The model under review builds one solid part; all positions refer to its coordinate system, in mm. Face numbers are marked on the shaded views. Coordinates: 2 decimals unless noted, no trailing zeros. Loops run counter-clockwise (first coordinate to the right, second up) from the corner with the lowest first, then second, coordinate; pieces in that order, holes last. Notation, with made-up numbers: M -1.5,70 L 13.5,70 A18 ccw 13.5,105 Z; hole C -9.75,-13 d1. An arc over 180 degrees is marked long. Use CSV: the item, a comma, the result in double quotes. Start each with the question number.
1. Draft analysis for pull direction Y (two halves, no side actions). For the marked faces 1, 2, 3 and 4, state which applies: +Y half, -Y half, draft (parallel to the pull), parting line (faces both ways), or undercut.
2. Clearance check with flat-ended pins moving along their axes: P1, Ø2, axis at x = 2, z = 5.5, coming from the +Y side; P2, Ø3, axis at y = -6.5, z = 1.5, coming from the +X side; P3, Ø1, axis at x = -30.5, y = 23, coming from the -Z side. State where each tip first meets the part, or that it passes through.
3. Add section A-A, the plane x = 0. Write out the cut boundary in (y, z), then the cut area to 3 significant figures.
4. Add section B-B, the plane z = 1.25. Write out the cut boundary in (x, y), then the cut area to 3 significant figures.
5. For L1, parallel to X at y = 1.5, z = 4; L2, parallel to X at y = 2, z = 5.5; L3, parallel to X at y = 23, z = 3, list the stretches that pass through material, from the lowest coordinate up.
6. Add section C-C, the plane y = 0. Write out the cut boundary in (x, z).
7. Add section D-D, the plane x = 27. Write out the cut boundary in (y, z), then the cut area to 3 significant figures.
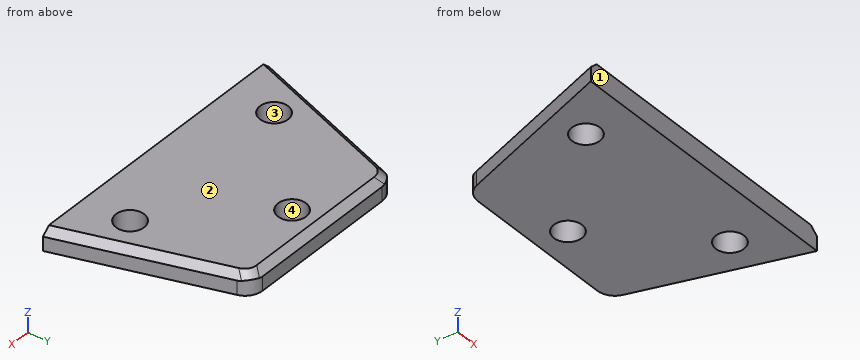
from build123d import *

# Parameters (mm, degrees)
F0_R     = 4
F1_DEPTH = 6
F2_SIZE  = 2
F3_F1_R  = 5
F3_F2_R  = 5
F3_F3_R  = 5
F3_F4_R  = 5


with BuildPart() as f1:
    # F0 (on Top) → F1 (new body)
    with BuildSketch(Plane.XY):
        Polygon((40.4508497187, -13.143277803), (25, 34.4095480118), (-25, 34.4095480118), (-40.4508497187, -13.143277803), align=None)
        with Locations((-25.7480759174, 0)):
            Circle(F0_R, mode=Mode.SUBTRACT)
        with Locations((25.7480759174, 0)):
            Circle(F0_R, mode=Mode.SUBTRACT)
        with Locations((0, 25.7480759174)):
            Circle(F0_R, mode=Mode.SUBTRACT)
    extrude(amount=F1_DEPTH)

    # F2
    f2_edges = [f1.edges().sort_by_distance(p)[0] for p in [
        (0, 34.409548, 6),
        (32.725425, 10.633135, 6),
        (-32.725425, 10.633135, 6),
    ]]
    chamfer(f2_edges, length=F2_SIZE)

    # F3: fillet of radius 5 on 4 edges, made by hand

    # F3_f1
    f3_f1_edges = [f1.edges().sort_by_distance(p)[0] for p in [
        (25, 34.4095480118, 2),
    ]]
    fillet(f3_f1_edges, radius=F3_F1_R)

    # F3_f2
    f3_f2_edges = [f1.edges().sort_by_distance(p)[0] for p in [
        (23.9265642827, 32.9320904977, 5.4774575141),
    ]]
    fillet(f3_f2_edges, radius=F3_F2_R)

    # F3_f3
    f3_f3_edges = [f1.edges().sort_by_distance(p)[0] for p in [
        (-25, 34.4095480118, 2),
    ]]
    fillet(f3_f3_edges, radius=F3_F3_R)

    # F3_f4
    f3_f4_edges = [f1.edges().sort_by_distance(p)[0] for p in [
        (-23.9265642827, 32.9320904977, 5.4774575141),
    ]]
    fillet(f3_f4_edges, radius=F3_F4_R)


solid = f1.part
Computed:
1,face 1,"-Y half"
1,face 2,"draft"
1,face 3,"undercut"
1,face 4,"undercut"
2,P1,"stops at y = 33.91"
2,P2,"stops at x = 38.78"
2,P3,"passes through"
3,outline,"M -13.14,0 L 21.75,0 L 21.75,6 L -13.14,6 Z; M 29.75,0 L 34.41,0 L 34.41,4 L 32.41,6 L 29.75,6 Z"
3,area,"235 mm^2"
4,outline,"M -40.45,-13.14 L 40.45,-13.14 L 26.12,30.95 A5 ccw 21.37,34.41 L -21.37,34.41 A5 ccw -26.12,30.95 Z; hole C -25.75,0 d8; hole C 0,25.75 d8; hole C 25.75,0 d8"
4,area,"2,960 mm^2"
5,L1,"x = -35.69 to -29.46, -22.04 to 22.04, 29.46 to 35.69"
5,L2,"x = -33.95 to -29.21, -22.28 to 22.28, 29.21 to 33.95"
5,L3,"x = -28.71 to -2.91, 2.91 to 28.71"
6,outline,"M -36.18,0 L -29.75,0 L -29.75,6 L -34.08,6 L -36.18,4 Z; M -21.75,0 L 21.75,0 L 21.75,6 L -21.75,6 Z; M 29.75,0 L 36.18,0 L 36.18,4 L 34.08,6 L 29.75,6 Z"
7,outline,"M -13.14,0 L -3.8,0 L -3.8,6 L -13.14,6 Z; M 3.8,0 L 28.25,0 L 28.25,4 L 21.78,6 L 3.8,6 Z"
7,area,"196 mm^2"
